Can you work these out from the model? Positions are in its coordinate system, mm. Face numbers are marked on the shaded views. A direction names the side the tool comes from. Coordinates: 2 decimals unless noted, no trailing zeros. Loops run counter-clockwise (first coordinate to the right, second up) from the corner with the lowest first, then second, coordinate; pieces in that order, holes last. Notation, with made-up numbers: (-6.5, -28) -> (21.5, -28) arc R18 ccw to (21.5, 2) -> close; hole circle Ø1 at (-30.75, -3.75). An arc over 180 degrees is marked (long way). Put each result on its own line as item: value. Start each with the question number.
Item 1: Please list where these lines run through material, in increasing order: L1, parallel to X at y = 25.75, z = 1.85; L2, parallel to X at y = 24.5, z = 0.6; L3, parallel to Y at x = 11.5, z = 0.5. Write a range as from..to.
Item 2: Will these pins go through, and if not, where does the flat tip stop? P1, Ø4, axis at x = 17.5, y = 24.5, coming from the +Z side; P2, Ø1.5, axis at y = 28.5, z = 2, coming from the -X side; P3, Ø1.5, axis at x = 29, z = 2, coming from the +Y side.
Item 3: We'd pull the mould along Y, two halves only. Please class the marked faces 1, 2, 3 and 4: pulls with the +Y half, pulls with the -Y half, needs draft (parallel to the pull), parting line crosses it, or undercut.
Item 4: If we section it at A-A on z = 0.7: Please give me the cut outline in (x, y).
Item 5: If we section it at C-C on x = 26.5: Please give me the cut outline in (y, z).
Item 6: If we section it at B-B on y = 20: Please give me the cut outline in (x, z), plus the area to 3 significant figures.
Item 7: For the marked faces 5 and 6, which set-ups out of +Z, -Z, +X, -X, +Y, -Y let a thin tool reach every point of the face, with its end or its side?
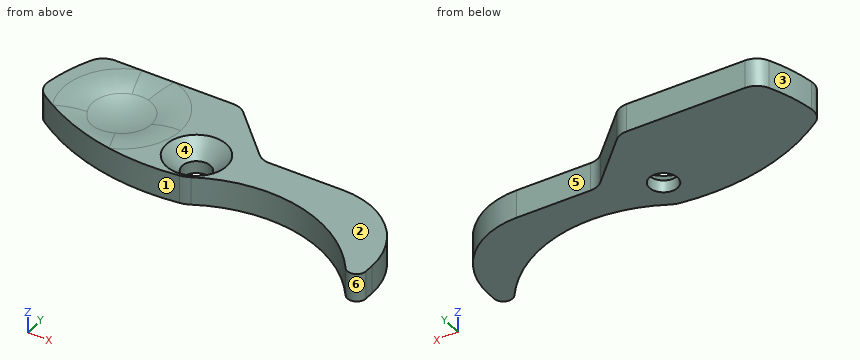
```python
from build123d import *

# Parameters (mm, degrees)
PAD003_DEPTH = 3
FILLET_R     = 10


with BuildPart() as sphere:
    # Sphere → Sphere (revolve)
    with BuildSketch(Plane(origin=(8, 27, 12), x_dir=(1, 0, 0), z_dir=(0, -1, 0))):
        with BuildLine():
            ThreePointArc((0, -10), (10, 0), (0, 10))
            Line((0, 10), (0, -10))
        make_face()
    revolve(axis=Axis((8, 27, 12), (0, 0, 1)))


with BuildPart() as clone_of_countersunk002:
    # Sketch007 → Revolution001 (revolve)
    with BuildSketch(Plane.YZ):
        Polygon((3.2, 0), (1.5, -1.7), (1.5, -10), (0, -10), (0, 0), align=None)
    revolve(axis=Axis((0, 0, 0), (0, 0, 1)))


with BuildPart() as clone_of_countersunk002_1:
    # Clone005 placement: moved
    add(clone_of_countersunk002.part.moved(Location((17.5, 24.5, 3))))


with BuildPart() as obj1:
    # Sketch → Pad003 (new body)
    with BuildSketch(Plane.XY):
        with BuildLine():
            ThreePointArc((17.903941, 21.027319), (18.426814, 21.146754), (18.920064, 21.357384))
            ThreePointArc((38.188772, 16.91527), (29.390013, 22.760914), (18.920064, 21.357384))
            ThreePointArc((38.188772, 16.91527), (39.30722, 16.548362), (40, 17.499993))
            Line((40, 18.499993), (40, 17.499993))
            ThreePointArc((40, 18.499993), (37.510407, 24.510406), (31.499995, 27))
            Line((23.656854, 27), (31.499995, 27))
            ThreePointArc((22.242641, 27.585786), (22.891487, 27.152241), (23.656854, 27))
            Line((22.242641, 27.585786), (17.414214, 32.414214))
            ThreePointArc((17.414214, 32.414214), (16.765367, 32.847759), (16, 33))
            Line((16, 33), (3.428753, 33))
            ThreePointArc((3.428753, 33), (2.351121, 32.684847), (1.613108, 31.83871))
            ThreePointArc((1.613108, 31.83871), (0.720961, 29.471304), (0.179492, 27))
            ThreePointArc((0.179492, 27), (0.325697, 25.914862), (1.021382, 25.069332))
            ThreePointArc((1.021382, 25.069332), (9.0844, 21.468416), (17.903941, 21.027319))
        make_face()
    extrude(amount=PAD003_DEPTH)

    # Cut003: cut Clone of Countersunk002
    add(clone_of_countersunk002_1.part, mode=Mode.SUBTRACT)

    # Cut004: cut Sphere
    add(sphere.part, mode=Mode.SUBTRACT)

    # Fillet
    fillet_edges = [obj1.edges().sort_by_distance(p)[0] for p in [
        (3.641101, 27, 3),
    ]]
    fillet(fillet_edges, radius=FILLET_R)


solid = obj1.part
```
Solutions:
1. L1: 0.41..15.88, 19.12..35.94
1. L2: 1.88..16, 19..37.52
1. L3: 21.02..33
2. P1: z = 1.8
2. P2: x = 0.3
2. P3: y = 27
3. face 1: pulls with the -Y half
3. face 2: needs draft
3. face 3: pulls with the +Y half
3. face 4: undercut
4. outline: (0.18, 27) arc R2 ccw to (1.02, 25.07) arc R24 ccw to (17.9, 21.03) arc R3 ccw to (18.92, 21.36) arc R15 cw to (38.19, 16.92) arc R1 ccw to (40, 17.5) -> (40, 18.5) arc R8.5 ccw to (31.5, 27) -> (23.66, 27) arc R2 cw to (22.24, 27.59) -> (17.41, 32.41) arc R2 ccw to (16, 33) -> (3.43, 33) arc R2 ccw to (1.61, 31.84) arc R17.5 ccw to start; hole circle Ø3 at (17.5, 24.5)
5. outline: (23.14, 0) -> (27, 0) -> (27, 3) -> (23.14, 3) -> close
6. outline: (35.21, 0) -> (39.87, 0) -> (39.87, 3) -> (35.21, 3) -> close
6. area: 14.0 mm^2
7. face 5: +Z, -Z, +X, +Y
7. face 6: +Z, -Z, -Y
